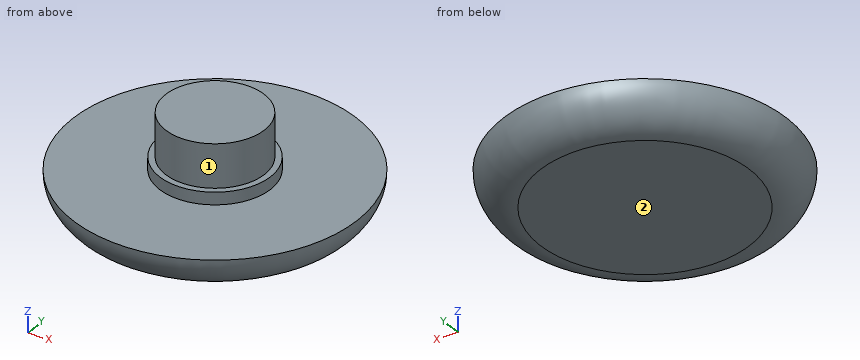
```python
from build123d import *

# Parameters (mm, degrees)
F0_R     = 4.5
F0_R_2   = 4.005
F1_DEPTH = 1
F2_DEPTH = 4.5
F0_R_3   = 11.5
F3_DEPTH = 3
F4_DEPTH = 3
F5_R     = 2.99999


# Not quite as in the source:
# - a fillet or chamfer is up to 0.001 mm smaller than in the source, because OpenCascade refuses the exact size


with BuildPart() as f1:
    # F0 (on Top) → F1 (new body)
    with BuildSketch(Plane.XY):
        Circle(F0_R)
        Circle(F0_R_2, mode=Mode.SUBTRACT)
    extrude(amount=F1_DEPTH)

    # F0 (on Top) → F2 (join)
    with BuildSketch(Plane.XY):
        Circle(F0_R_2)
    extrude(amount=F2_DEPTH)

    # F0 (on Top) → F3 (join)
    with BuildSketch(Plane.XY):
        Circle(F0_R_3)
        Circle(F0_R, mode=Mode.SUBTRACT)
    extrude(amount=-F3_DEPTH)

    # F0 (on Top) → F4 (join)
    with BuildSketch(Plane.XY):
        Circle(F0_R)
        Circle(F0_R_2, mode=Mode.SUBTRACT)
        Circle(F0_R_2)
    extrude(amount=-F4_DEPTH)

    # F5 (radius 3 in the source; OpenCascade refuses exactly that, so slightly less here)
    f5_edges = [f1.edges().sort_by_distance(p)[0] for p in [
        (-11.5, 0, -3),
    ]]
    fillet(f5_edges, radius=F5_R)


solid = f1.part
```
Could you check a few things on this model? Use its own coordinates, in mm. Face numbers are marked on the shaded views. A direction names the side the tool comes from. Round coordinates to 2 decimals unless told otherwise and drop trailing zeros. Loops run counter-clockwise (first coordinate to the right, second up) from the corner with the lowest first, then second, coordinate; pieces in that order, holes last.
Q1. I want a section at B-B (z = 2.5). Write out the boundary of the cut face in (x, y) (3 decimals).
Q2. I want a section at C-C (z = -2.25). Write out the boundary of the cut face in (x, y), and give its area (3 significant figures).
Q3. For P1, Ø1, axis at y = 0, z = -1, coming from the +X side; P2, Ø1, axis at x = 6.5, y = 6.5, coming from the -Z side; P3, Ø3, axis at y = 3.5, z = -0.5, coming from the +X side, each with a flat end and sliding along its axis, tell me the tip position at first contact or that it passes through.
Q4. On a 3-axis mill with a long thin cutter (end or side, diameter ignored), from which of +Z, -Z, +X, -X, +Y, -Y can I reach the whole of each face in a straight line? I mean the marked faces 1 and 2. Say none if no direction works.
Q5. Please list where these lines run through material, in increasing order: L1, parallel to Z at x = -3.25, y = -7; L2, parallel to Y at x = -1.75, z = -1.25; L3, parallel to Y at x = 1.5, z = 3.
Answer below:
1. outline: circle Ø8.01 at (0, 0)
2. outline: circle Ø20.97 at (0, 0)
2. area: 345 mm2
3. P1: stops at x = 11.46
3. P2: stops at z = -2.99
3. P3: stops at x = 11.31
4. face 1: +Z
4. face 2: -Z, +X, -X, +Y, -Y
5. L1: z = -3 to 0
5. L2: y = -11.09 to 11.09
5. L3: y = -3.71 to 3.71
